```python
from build123d import *

# Parameters (mm, degrees)
BOSS_EXTRUDE1_DEPTH = 3.175
SKETCH2_W           = 3.175
SKETCH2_H           = 44.45
CUT_EXTRUDE1_DEPTH  = 3.175


with BuildPart() as part:
    # Sketch1 → Boss-Extrude1 (new body)
    with BuildSketch(Plane(origin=(0, 0, 0), x_dir=(1, 0, 0), z_dir=(0, 1, 0))):
        Polygon((-41.275, -19.05), (-41.275, 19.05), (-44.45, 19.05), (-44.45, 31.75), (-41.275, 31.75), (41.275, 31.75), (44.45, 31.75), (44.45, 19.05), (41.275, 19.05), (41.275, -19.05), (44.45, -19.05), (44.45, -31.75), (41.275, -31.75), (-41.275, -31.75), (-44.45, -31.75), (-44.45, -19.05), align=None)
    extrude(amount=BOSS_EXTRUDE1_DEPTH)

    # Sketch2 → Cut-Extrude1 (cut)
    with BuildSketch(Plane(origin=(0, 3.175, 0), x_dir=(1, 0, 0), z_dir=(0, 1, 0))):
        Rectangle(SKETCH2_W, SKETCH2_H)
    extrude(amount=-CUT_EXTRUDE1_DEPTH, mode=Mode.SUBTRACT)


solid = part.part
```
Model file for the job. Use its own axes, mm. A direction names the side the tool comes from. Coordinates: 2 decimals unless noted, no trailing zeros. Loops run counter-clockwise (first coordinate to the right, second up) from the corner with the lowest first, then second, coordinate; pieces in that order, holes last. Notation, with made-up numbers: (57.5, -29.5) - (110.5, -29.5) arc R29 ccw to (110.5, 0.5) - close; hole circle Ø11 at (15, 84). An arc over 180 degrees is marked (long way). Write item = value, one per line. Start each with the question number.
Item 1: 3-axis set-ups, long thin cutter, end or side, ignore diameter. For faces 1 (the face through (-43, 2, 19.05)), 2 (the face through (0, 2, 22.225)), 3 (the face through (43, 2, 19.05)): which of +Z, -Z, +X, -X, +Y, -Y reach the whole face in a straight line?
Item 2: Drop flat-ended pins along their axis: pin 1 Ø1.6 at (y, z) = (2, 5.5) entering from +X (3 decimals); pin 2 Ø1 at (y, z) = (1.5, 10.5) entering from -X (3 decimals). Give the stop position or say it passes through.
Item 3: Pull direction Z, two halves, no side cores. Call faces 4 (the face through (-1, 2, 31.75)), 5 (the face through (-44.45, 2, -25)), 6 (the face through (-43, 2, -19.05)): +Z half, -Z half, draft (parallel to the pull), parting line (faces both ways), or undercut.
Item 4: Saw through at C-C, the plane z = 7. List the corners of the cut face in (x, y) (1 decimal).
Item 5: Wall check: probe 1 along X at (y, z) = (0.35, -17.5) (1 decimal); probe 2 along X at (y, z) = (1.5, 20); probe 3 along Z at (x, y) = (-1, 0.7) (3 decimals). Give the ranges that are in metal, low to high. Write a range as [from, to].
Answers:
q1.face_1 = -X, +Y, -Y
q1.face_2 = +Y, -Y
q1.face_3 = +X, +Y, -Y
q2.pin_1 = 41.275
q2.pin_2 = -41.275
q3.face_4 = +Z half
q3.face_5 = draft
q3.face_6 = undercut
q4.outline = (-41.3, 0) - (-1.6, 0) - (-1.6, 3.2) - (-41.3, 3.2) - close; (1.6, 0) - (41.3, 0) - (41.3, 3.2) - (1.6, 3.2) - close
q5.probe_1 = [-41.3, -1.6], [1.6, 41.3]
q5.probe_2 = [-44.45, -1.59], [1.59, 44.45]
q5.probe_3 = [-31.75, -22.225], [22.225, 31.75]
